```python
from build123d import *

# Parameters (mm, degrees)
BOSS_EXTRUDE1_DEPTH   = 2.5
SKETCH1_R             = 7.4
BOSS_EXTRUDE1_2_DEPTH = 2.5
BOSS_EXTRUDE4_START   = -10
BOSS_EXTRUDE4_DEPTH   = 14
SKETCH2_W             = 5
SKETCH2_H             = 25.381176
CUT_EXTRUDE1_DEPTH    = 20
CUT_EXTRUDE2_DEPTH    = 4
SKETCH4_R             = 2.1
CUT_EXTRUDE3_DEPTH    = 87.16844


# Read off the part's stored shape, not the designer's step: Boss-Extrude4
with BuildPart() as part:
    # Sketch1 → Boss-Extrude1 (new, symmetric)
    with BuildSketch(Plane.XY):
        with BuildLine():
            Line((-9.998498, 74.826667), (-7.698412, -57.850642))
            Line((-7.698412, -57.850642), (7.698412, -57.850642))
            Line((7.698412, -57.850642), (9.998498, 74.826667))
            ThreePointArc((9.998498, 74.826667), (0, 85), (-9.998498, 74.826667))
        make_face()
    extrude(amount=BOSS_EXTRUDE1_DEPTH, both=True)



with BuildPart() as body_2:
    # Sketch1 → Boss-Extrude1 2 (new, symmetric)
    with BuildSketch(Plane.XY):
        with Locations((0, -75)):
            Circle(SKETCH1_R)
    extrude(amount=BOSS_EXTRUDE1_2_DEPTH, both=True)


with BuildPart() as part_1:
    add(part.part)

    add(body_2.part)  # Boss-Extrude4 merges body 2
    # Boss-Extrude4 outline → Boss-Extrude4 (add)
    with BuildSketch(Plane.XY.offset(BOSS_EXTRUDE4_START)):
        with BuildLine():
            Line((-7.698412, -57.850642), (-7.398888, -75.128267))
            ThreePointArc((-7.398888, -75.128267), (0, -82.4), (7.398888, -75.128267))
            Line((7.398888, -75.128267), (7.698412, -57.850642))
            Line((7.698412, -57.850642), (-7.698412, -57.850642))
        make_face()
    extrude(amount=BOSS_EXTRUDE4_DEPTH)

    # Sketch2 → Cut-Extrude1 (cut)
    with BuildSketch(Plane(origin=(-8.698693, -0.1508, 0), x_dir=(0, 0, 1), z_dir=(-0.9998497664927245, -0.017333333333333607, 0))):
        with Locations((-1, -72.965255)):
            Rectangle(SKETCH2_W, SKETCH2_H)
    extrude(amount=-CUT_EXTRUDE1_DEPTH, mode=Mode.SUBTRACT)

    # Sketch3 → Cut-Extrude2 (cut)
    with BuildSketch(Plane(origin=(0, 0, -10), x_dir=(-1, 0, 0), z_dir=(0, 0, -1))):
        with BuildLine():
            Line((-7.698412, -57.850642), (-7.398888, -75.128267))
            ThreePointArc((-7.398888, -75.128267), (-0.064136, -67.600278), (7.4, -75))
            ThreePointArc((7.4, -75), (7.399722, -75.064136), (7.398888, -75.128267))
            Line((7.398888, -75.128267), (7.698412, -57.850642))
            Line((7.698412, -57.850642), (-7.698412, -57.850642))
        make_face()
        with BuildLine():
            ThreePointArc((7.4, -75), (-0.064136, -67.600278), (-7.398888, -75.128267))
            ThreePointArc((-7.398888, -75.128267), (0, -82.4), (7.398888, -75.128267))
            ThreePointArc((7.398888, -75.128267), (7.399722, -75.064136), (7.4, -75))
        make_face()
    extrude(amount=-CUT_EXTRUDE2_DEPTH, mode=Mode.SUBTRACT)

    # Sketch4 → Cut-Extrude3 (cut, through all)
    with BuildSketch(Plane.XY.offset(4)):
        with Locations((0, 75)):
            Circle(SKETCH4_R)
        with Locations((0, -75)):
            Circle(SKETCH4_R)
    extrude(amount=-CUT_EXTRUDE3_DEPTH, mode=Mode.SUBTRACT)


solid = part_1.part
```
Design review of the part built by this model. Coordinates are the model's own, in mm. A direction names the side the tool comes from. Round coordinates to 2 decimals unless told otherwise and drop trailing zeros. Write each loop counter-clockwise with the first axis right and the second up, starting at its lowest first coordinate (ties: lowest second). Pieces come first, ordered by that corner, then holes. Notation, with made-up numbers: (54.25, -32.5) -> (105.25, -32.5) arc R33 cw to (105.25, -3.5) -> close; hole circle Ø4 at (30.5, 89). An arc over 180 degrees is marked (long way). Write item = value, one per line. Start each with the question number.
1) Tool access review of faces 1 (the face through (0, -70, -6)), 2 (the face through (0, 15, 2.5)), 3 (the face through (0, 15, -2.5)): name each direction out of +Z, -Z, +X, -X, +Y, -Y from which nothing blocks a thin tool from reaching the whole face with its end or side.
2) Wall thickness on probe 1 along Y at (x, z) = (0, -4.35); probe 2 along Z at (x, y) = (4.5, 15); probe 3 along Y at (x, z) = (1.5, -5): over which ranges is each line inside the solid? List them lowest first. Write a range as from..to.
3) Mouldability with a two-part tool opening along Y and no side actions: class faces 4 (the face through (0, -71, -3.5)), 5 (the face through (-0.16, -82.4, -4.77)), 6 (the face through (1.13, 76.77, 0.04)) as +Y half, -Y half, draft (parallel to the pull), parting line (faces both ways), or undercut.
4) Take a section at C-C, the plane x = 6. State the section outline as (y, z) points.
5) Clearance check with flat-ended pins moving along their axes: pin 1 (6 mm diameter, centred on x = -4.5, y = 45.5, fed in from +Z); pin 2 (6 mm diameter, centred on x = 7, z = -1, fed in from -Y); pin 3 (5 mm diameter, centred on y = -43.5, z = -4, fed in from +X). State where each tip first meets the part, or that it passes through.
6) Take a section at B-B, the plane x = 0. State the section outline as (y, z) points, plus the area to 3 significant figures.
7) Take a section at A-A, the plane z = 0. State the section outline as (x, y) points, plus the area to 3 significant figures.
8) Take a section at D-D, the plane y = -9.5. State the section outline as (x, z) points.
Results list:
q1.face_1 = -Z, +X, -X, +Y, -Y
q1.face_2 = +Z, +X, -X, +Y
q1.face_3 = -Z, +X, -X, +Y
q2.probe_1 = -82.4..-77.1, -72.9..-57.85
q2.probe_2 = -2.5..2.5
q2.probe_3 = -82.25..-76.47, -73.53..-57.85
q3.face_4 = draft
q3.face_5 = -Y half
q3.face_6 = undercut
q4.outline = (-79.33, -6) -> (-57.85, -6) -> (-57.85, -2.5) -> (83, -2.5) -> (83, 2.5) -> (-57.85, 2.5) -> (-57.85, 4) -> (-79.33, 4) -> (-79.33, 1.5) -> (-60.18, 1.5) -> (-60.18, -3.5) -> (-79.33, -3.5) -> close
q5.pin_1 = 2.5
q5.pin_2 = -80.12
q5.pin_3 = 7.98
q6.outline = (-82.4, -6) -> (-77.1, -6) -> (-77.1, -3.5) -> (-82.4, -3.5) -> close; (-82.4, 1.5) -> (-77.1, 1.5) -> (-77.1, 4) -> (-82.4, 4) -> close; (-72.9, -6) -> (-57.85, -6) -> (-57.85, -2.5) -> (72.9, -2.5) -> (72.9, 2.5) -> (-57.85, 2.5) -> (-57.85, 4) -> (-72.9, 4) -> (-72.9, 1.5) -> (-60.28, 1.5) -> (-60.28, -3.5) -> (-72.9, -3.5) -> close; (77.1, -2.5) -> (85, -2.5) -> (85, 2.5) -> (77.1, 2.5) -> close
q6.area = 807 mm²
q7.outline = (-10, 74.83) -> (-7.65, -60.42) -> (7.66, -60.15) -> (10, 74.83) arc R10 ccw (long way) to start; hole circle Ø4.2 at (0, 75)
q7.area = 2,530 mm²
q8.outline = (-8.54, -2.5) -> (8.54, -2.5) -> (8.54, 2.5) -> (-8.54, 2.5) -> close
